Geometry: final body of the model. Coordinates: model frame, mm. Face numbers are marked on the shaded views. A direction names the side the tool comes from. Coordinates: 2 decimals unless noted, no trailing zeros. Write each loop counter-clockwise with the first axis right and the second up, starting at its lowest first coordinate (ties: lowest second). Pieces come first, ordered by that corner, then holes.
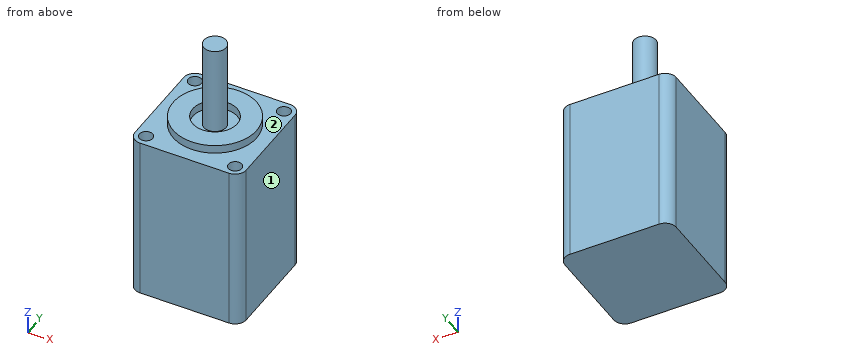
from build123d import *

# Parameters (mm, degrees)
BOSS_EXTRUDE1_DEPTH      = 30
SKETCH3_R                = 7.5
SKETCH3_R_2              = 4
BOSS_EXTRUDE2_DEPTH      = 1.5
SKETCH4_R                = 2
BOSS_EXTRUDE3_DEPTH      = 16
M2_CLEARANCE_HOLE1_D     = 2.4
M2_CLEARANCE_HOLE1_DEPTH = 3.5
M2_CLEARANCE_HOLE1_TIP   = 0.721032743


with BuildPart() as part:
    # Sketch1 → Boss-Extrude1 (new body)
    with BuildSketch(Plane.XY):
        with BuildLine():
            Line((-8, -10), (8, -10))
            ThreePointArc((8, -10), (9.414213562, -9.414213562), (10, -8))
            Line((10, -8), (10, 8))
            ThreePointArc((10, 8), (9.414213562, 9.414213562), (8, 10))
            Line((8, 10), (-8, 10))
            ThreePointArc((-8, 10), (-9.414213562, 9.414213562), (-10, 8))
            Line((-10, 8), (-10, -8))
            ThreePointArc((-10, -8), (-9.414213562, -9.414213562), (-8, -10))
        make_face()
    extrude(amount=-BOSS_EXTRUDE1_DEPTH)

    # Sketch3 → Boss-Extrude2 (add)
    with BuildSketch(Plane.XY):
        Circle(SKETCH3_R)
        Circle(SKETCH3_R_2, mode=Mode.SUBTRACT)
    extrude(amount=BOSS_EXTRUDE2_DEPTH)

    # Sketch4 → Boss-Extrude3 (add)
    with BuildSketch(Plane.XY):
        Circle(SKETCH4_R)
    extrude(amount=BOSS_EXTRUDE3_DEPTH)

    # M2 Clearance Hole1
    with Locations(Plane.XY):
        with Locations((-8, 8), (8, 8), (8, -8), (-8, -8)):
            Hole(M2_CLEARANCE_HOLE1_D / 2, depth=M2_CLEARANCE_HOLE1_DEPTH)
            with Locations((0, 0, -(M2_CLEARANCE_HOLE1_DEPTH + M2_CLEARANCE_HOLE1_TIP / 2))):  # 118° drill point
                Cone(0, M2_CLEARANCE_HOLE1_D / 2, M2_CLEARANCE_HOLE1_TIP, mode=Mode.SUBTRACT)


solid = part.part
Item 1: Section A-A, the plane y = 6. Output: boundary loops of the cut face in (x, z).
Derived:
outline: (-10, -30) - (10, -30) - (10, 0) - (4.5, 0) - (4.5, 1.5) - (-4.5, 1.5) - (-4.5, 0) - (-10, 0) - close
Item 2: Section D-D, the plane x = -6.25. Output: boundary loops of the cut face in (y, z).
Derived:
outline: (-10, -30) - (10, -30) - (10, 0) - (4.15, 0) - (4.15, 1.5) - (-4.15, 1.5) - (-4.15, 0) - (-10, 0) - close
Item 3: Pin query (flat end, axial travel): pin 1 (3 mm diameter, centred on x = 8, y = 8, fed in from +Z); pin 2 (5 mm diameter, centred on x = -2.5, z = 7.5, fed in from -Y); pin 3 (1.9 mm diameter, centred on x = -8, y = 8, fed in from +Z); pin 4 (10 mm diameter, centred on x = 4, y = -4, fed in from +Z). Return the tip coordinate at first contact, or that it passes through.
Derived:
pin 1: stops at z = 0
pin 2: stops at y = -2
pin 3: stops at z = -3.65
pin 4: stops at z = 16
Item 4: Set-up query: the marked faces 1 and 2. Return all of +Z, -Z, +X, -X, +Y, -Y with unobstructed straight access to the full face (end or side cutting, diameter ignored); none if empty.
Derived:
face 1: +Z, -Z, +X, +Y, -Y
face 2: +Z
Item 5: Material intervals for probe 1 along Y at (x, z) = (8, -0.95); probe 2 along Y at (x, z) = (0, 0.95), sorted ascending.
Derived:
probe 1: y = -10 to -9.2, -6.8 to 6.8, 9.2 to 10
probe 2: y = -7.5 to -4, -2 to 2, 4 to 7.5
Item 6: Section C-C, the plane z = 3. Output: boundary loops of the cut face in (x, y).
Derived:
outline: circle Ø4 at (0, 0)
Item 7: Section B-B, the plane x = 0. Output: boundary loops of the cut face in (y, z), plus the area to 4 significant figures.
Derived:
outline: (-10, -30) - (10, -30) - (10, 0) - (7.5, 0) - (7.5, 1.5) - (4, 1.5) - (4, 0) - (2, 0) - (2, 16) - (-2, 16) - (-2, 0) - (-4, 0) - (-4, 1.5) - (-7.5, 1.5) - (-7.5, 0) - (-10, 0) - close
area: 674.5 mm2
